Part print with two shaded views. Sizes in mm from the minimum x, y, z corner. A direction names the side the tool comes from. Round coordinates to 2 decimals unless told otherwise and drop trailing zeros. Loops run counter-clockwise (first coordinate to the right, second up) from the corner with the lowest first, then second, coordinate; pieces in that order, holes last.
(1) Cut at A-A on y = 5.75. List the corners of the cut face in (x, z).
(2) Cut at B-B on x = 10.25. List the corners of the cut face in (y, z) (3 decimals).
(3) Cut at C-C on z = 15.25. List the corners of the cut face in (x, y).
(4) Mould opens along X. For the marked faces 3, 4, 5 and 6 say: +X half, -X half, draft (parallel to the pull), parting line (faces both ways), or undercut.
(5) Flat gauge pins, fed straight in: pin 1 (1 mm diameter, centred on x = 10.5, y = 3.5, fed in from -Z); pin 2 (1.5 mm diameter, centred on x = 8, z = 4.5, fed in from +Y). Where does each tip first touch, or does it go through?
(6) Cut at D-D on z = 8. List the corners of the cut face in (x, y), then the cut area to 3 significant figures.
(7) Probe probe 1 along X at (y, z) = (9, 8); probe 2 along Z at (x, y) = (10.25, 1.5) (3 decimals); probe 3 along X at (y, z) = (9.75, 11.25). List the from-to ranges inside material, lowest first.
(8) Tool access for the marked faces 1 and 2: list every direction of +Z, -Z, +X, -X, +Y, -Y with a clear straight run to the whole face (end or side of a thin tool).
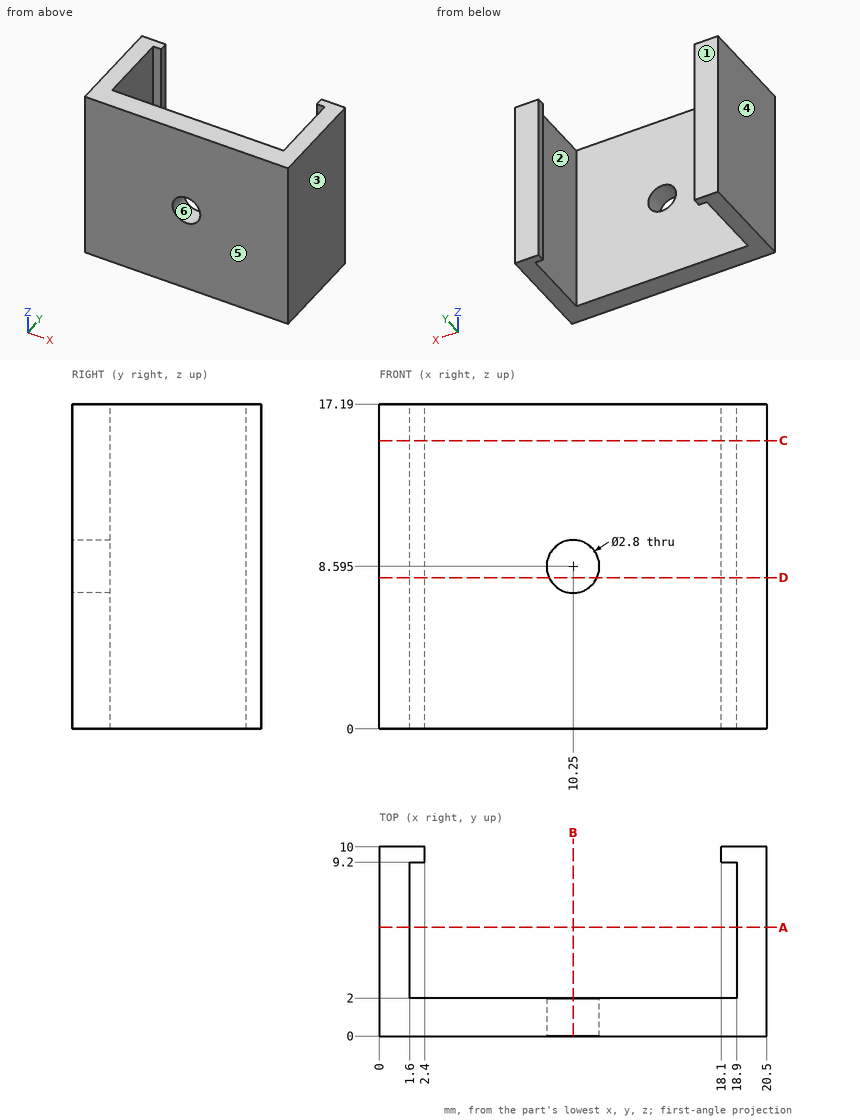
Final values:
1. outline: (0, 0) - (1.6, 0) - (1.6, 17.19) - (0, 17.19) - close; (18.9, 0) - (20.5, 0) - (20.5, 17.19) - (18.9, 17.19) - close
2. outline: (0, 0) - (2, 0) - (2, 7.195) - (0, 7.195) - close; (0, 9.995) - (2, 9.995) - (2, 17.19) - (0, 17.19) - close
3. outline: (0, 0) - (20.5, 0) - (20.5, 10) - (18.1, 10) - (18.1, 9.2) - (18.9, 9.2) - (18.9, 2) - (1.6, 2) - (1.6, 9.2) - (2.4, 9.2) - (2.4, 10) - (0, 10) - close
4. face 3: +X half
4. face 4: -X half
4. face 5: draft
4. face 6: undercut
5. pin 1: passes through
5. pin 2: stops at y = 2
6. outline: (0, 0) - (8.98, 0) - (8.98, 2) - (1.6, 2) - (1.6, 9.2) - (2.4, 9.2) - (2.4, 10) - (0, 10) - close; (11.52, 0) - (20.5, 0) - (20.5, 10) - (18.1, 10) - (18.1, 9.2) - (18.9, 9.2) - (18.9, 2) - (11.52, 2) - close
6. area: 62.8 mm2
7. probe 1: x = 0 to 1.6, 18.9 to 20.5
7. probe 2: z = 0 to 7.195, 9.995 to 17.19
7. probe 3: x = 0 to 2.4, 18.1 to 20.5
8. face 1: +Z, -Z, +X, -X, +Y
8. face 2: +Z, -Z
